Can you work these out from the model? Positions are in its coordinate system, mm. A direction names the side the tool comes from. Give positions to 0.01 mm unless a question says otherwise; leave off trailing zeros. Order: outer loops, then holes, each group sorted by start corner. A loop starts at its lowest first (then second) coordinate and runs counter-clockwise, first axis right, second up.
Item 1: I want a section at A-A, the plane z = 15. Write out the boundary of the cut face in (x, y).
Item 2: I want a section at B-B, the plane y = 21. Write out the boundary of the cut face in (x, z).
Item 3: Which directions (+Z, -Z, +X, -X, +Y, -Y) give clear straight access to the entire face, cutting with the end or side of a thin tool? Please do faces 1 (the flat face through (17.8, -43.376, -12.522)), 2 (the flat face through (-18.178, -43.175, -12.522)), 3 (the flat face through (17.709, -43.465, 125.222)), 4 (the flat face through (18.212, 43.256, 125.222)).
Item 4: I'm going to push flat-ended pins straight in: pin 1 Ø4 at (x, z) = (2.5, 42) entering from -Y; pin 2 Ø10 at (x, z) = (-24, 214) entering from -Y; pin 3 Ø12 at (x, z) = (11.5, 46.5) entering from +Y; pin 4 Ø12 at (x, y) = (34.5, 40) entering from -Z. Where does each tip first touch, or does it pass through?
Item 5: If I drill on line 1 along X through (y, z) = (0, 58); line 2 along X through (y, z) = (19, 156.5); line 3 along Y through (x, z) = (-19.5, 201.5), over which ranges is the centre line in solid material (lowest first)?
```python
from build123d import *

# Parameters (mm, degrees)
F1_DEPTH = 254
F3_DEPTH = 25.4


with BuildPart() as f1:
    # F0 (on Top) → F1 (new body)
    with BuildSketch(Plane.XY):
        Polygon((35.921024, -35.921024), (50.8, 0), (35.921024, 35.921024), (0, 50.8), (-35.921024, 35.921024), (-50.8, 0), (-35.921024, -35.921024), (0, -50.8), align=None)
    extrude(amount=F1_DEPTH)

    # F2 (on Top) → F3 (join)
    with BuildSketch(Plane.XY):
        Polygon((-50.949764, 0), (-35.853539, -36.105141), (0, 0), align=None)
        Polygon((0, 0), (-35.853539, -36.105141), (0, -50.446555), align=None)
        Polygon((36.105141, -36.105141), (0, 0), (0, -50.446555), align=None)
        Polygon((-50.949764, 0), (0, 0), (-35.853539, 36.105141), align=None)
        Polygon((-35.853539, 36.105141), (0, 0), (0, 50.698161), align=None)
        Polygon((0, 50.698161), (0, 0), (36.105141, 36.105141), align=None)
        Polygon((51.201366, 0), (0, 0), (36.105141, -36.105141), align=None)
        Polygon((36.105141, 36.105141), (0, 0), (51.201366, 0), align=None)
    extrude(amount=-F3_DEPTH)


solid = f1.part
```
Results list:
1. outline: (-50.8, 0) - (-35.92, -35.92) - (0, -50.8) - (35.92, -35.92) - (50.8, 0) - (35.92, 35.92) - (0, 50.8) - (-35.92, 35.92) - close
2. outline: (-42.17, -25.4) - (42.42, -25.4) - (42.42, 0) - (42.1, 0) - (42.1, 254) - (-42.1, 254) - (-42.1, 0) - (-42.17, 0) - close
3. face 1: -Z, +X, -Y
3. face 2: -Z, -X, -Y
3. face 3: +Z, +X, -Y
3. face 4: +Z, +X, +Y
4. pin 1: stops at y = -50.59
4. pin 2: stops at y = -42.93
4. pin 3: stops at y = 48.52
4. pin 4: stops at z = -25.4
5. line 1: x = -50.8 to 50.8
5. line 2: x = -42.93 to 42.93
5. line 3: y = -42.72 to 42.72
